from build123d import *

# Parameters (mm, degrees)
BOSS_EXTRU_1_DEPTH      = 8
ESQUISSE2_R             = 0.5
ENL_V_MAT_EXTRU_1_DEPTH = 8


with BuildPart() as part:
    # Esquisse1 → Boss.-Extru.1 (new body)
    with BuildSketch(Plane.XY):
        with BuildLine():
            Line((-114.826935211, -6.347820711), (-114.826935211, -44.347820711))
            Line((-114.826935211, -44.347820711), (-60.826935211, -44.347820711))
            Line((-60.826935211, -44.347820711), (-60.826935211, -6.347820711))
            Line((-60.826935211, -6.347820711), (-70.826935211, -6.347820711))
            Line((-70.826935211, -6.347820711), (-70.826935211, -12.226500367))
            ThreePointArc((-70.826935211, -12.226500367), (-70.826935211, -14.347820711), (-72.948255555, -14.347820711))
            Line((-72.948255555, -14.347820711), (-102.705614868, -14.347820711))
            ThreePointArc((-102.705614868, -14.347820711), (-104.826935211, -14.347820711), (-104.826935211, -12.226500367))
            Line((-104.826935211, -12.226500367), (-104.826935211, -6.347820711))
            Line((-104.826935211, -6.347820711), (-114.826935211, -6.347820711))
        make_face()
    extrude(amount=BOSS_EXTRU_1_DEPTH)

    # Esquisse2 → Enlèv. mat.-Extru.1 (cut)
    with BuildSketch(Plane.XY.offset(8)):
        with Locations((-110.826935211, -18.347820711)):
            Circle(ESQUISSE2_R)
        with Locations((-64.826935211, -18.347820711)):
            Circle(ESQUISSE2_R)
        with Locations((-64.826935211, -40.347820711)):
            Circle(ESQUISSE2_R)
        with Locations((-110.826935211, -40.347820711)):
            Circle(ESQUISSE2_R)
    extrude(amount=-ENL_V_MAT_EXTRU_1_DEPTH, mode=Mode.SUBTRACT)


solid = part.part
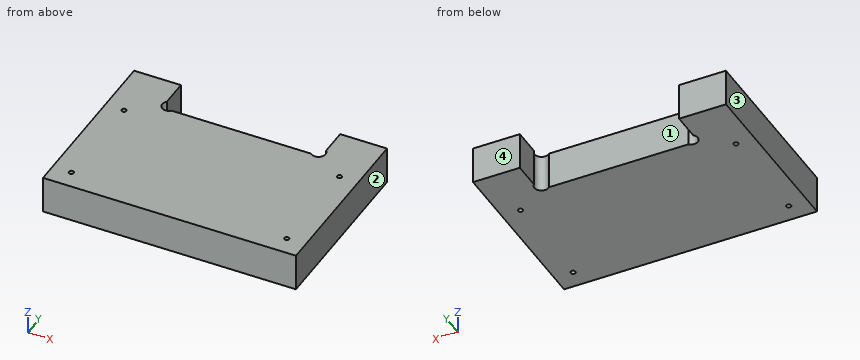
Design review of the part built by this model. Coordinates are the model's own, in mm. Face numbers are marked on the shaded views. Coordinates: 2 decimals unless noted, no trailing zeros. Order: outer loops, then holes, each group sorted by start corner. A loop starts at its lowest first (then second) coordinate and runs counter-clockwise, first axis right, second up. Notation, with made-up numbers: (62, 65.25) -> (111, 65.25) arc R24 cw to (111, 76.25) -> close; hole circle Ø5 at (45, 64). An arc over 180 degrees is marked (long way). One line per item, written item: value.
1) We need section B-B, the plane z = 6. Give the boundary of the cut face in (x, y).
Output values:
outline: (-114.83, -44.35) -> (-60.83, -44.35) -> (-60.83, -6.35) -> (-70.83, -6.35) -> (-70.83, -12.23) arc R1.5 cw to (-72.95, -14.35) -> (-102.71, -14.35) arc R1.5 cw to (-104.83, -12.23) -> (-104.83, -6.35) -> (-114.83, -6.35) -> close; hole circle Ø1 at (-110.83, -40.35); hole circle Ø1 at (-110.83, -18.35); hole circle Ø1 at (-64.83, -40.35); hole circle Ø1 at (-64.83, -18.35)
2) We need section A-A, the plane y = -10.5. Give the boundary of the cut face in (x, z).
Output values:
outline: (-114.83, 0) -> (-104.83, 0) -> (-104.83, 8) -> (-114.83, 8) -> close; (-70.83, 0) -> (-60.83, 0) -> (-60.83, 8) -> (-70.83, 8) -> close
3) We need section C-C, the plane x = -99.5. Give the boundary of the cut face in (y, z), then the cut area to 3 significant figures.
Output values:
outline: (-44.35, 0) -> (-14.35, 0) -> (-14.35, 8) -> (-44.35, 8) -> close
area: 240 mm2
4) Clearance check with flat-ended pins moving along their axes: P1, Ø2.5, axis at x = -95, z = 4.5, coming from the +Y side; P2, Ø6, axis at x = -105, y = -19, coming from the -Z side. State where each tip first meets the part, or that it passes through.
Output values:
P1: stops at y = -14.35
P2: stops at z = 0
5) To check wall thickness, follow probe 1 along X at (y, z) = (-18, 5.75); probe 2 along X at (y, z) = (-9.5, 4.75); probe 3 along Y at (x, z) = (-82.5, 6.5). State the ranges of each line that lie inside material, in increasing order. Write a range as [from, to].
Output values:
probe 1: x = [-114.83, -111.19], [-110.47, -65.19], [-64.47, -60.83]
probe 2: x = [-114.83, -104.83], [-70.83, -60.83]
probe 3: y = [-44.35, -14.35]
6) Draft analysis for pull direction X (two halves, no side actions). For the marked faces 1, 2, 3 and 4, state which applies: +X half, -X half, draft (parallel to the pull), parting line (faces both ways), or undercut.
Output values:
face 1: undercut
face 2: +X half
face 3: -X half
face 4: draft
